Work out the finished part from the listing and answer in its coordinate system (mm). Give positions to 0.01 mm unless a question says otherwise; leave off trailing zeros. Write each loop counter-clockwise with the first axis right and the second up, starting at its lowest first coordinate (ties: lowest second). Pieces come first, ordered by that corner, then holes.
1) Given pin 1 Ø0.9 at (x, z) = (-64.5, 2) entering from +Y, flat-ended and moving along its own axis, determine where the tip first touches the part or whether it passes through.
2) Straight lines are drawn through the part: probe 1 along X at (y, z) = (17.5, 0.2); probe 2 along Y at (x, z) = (-15, 2.15); probe 3 along X at (y, z) = (-11, 1). For each, find the intervals that lie inside material, in ascending order.
3) Find section A-A (x = 8). Determine the outline of the cut face in (y, z).
4) Find section B-B (z = 1.5). Count the separate pieces of the cut face and the enclosed holes in it, plus the area to 3 significant figures.
```python
from build123d import *

# Parameters (mm, degrees)
SKETCH1_R           = 1.42
SKETCH1_W           = 25.000092503
SKETCH1_H           = 60
SKETCH1_W_2         = 30
SKETCH1_H_2         = 30
SKETCH1_W_3         = 20
SKETCH1_H_3         = 1
BOSS_EXTRUDE1_DEPTH = 3


with BuildPart() as part:
    # Sketch1 → Boss-Extrude1 (new body)
    with BuildSketch(Plane.XY):
        Polygon((-55, 45), (45, 45), (45, -45), (-55, -45), (-55, -30), (-140, -30), (-140, 30), (-55, 30), align=None)
        with Locations((15, 39)):
            Circle(SKETCH1_R, mode=Mode.SUBTRACT)
        with Locations((-15, 39)):
            Circle(SKETCH1_R, mode=Mode.SUBTRACT)
        with Locations((-15, -39)):
            Circle(SKETCH1_R, mode=Mode.SUBTRACT)
        with Locations((15, -39)):
            Circle(SKETCH1_R, mode=Mode.SUBTRACT)
        with Locations((30.000092503, 39.056338633)):
            Circle(SKETCH1_R, mode=Mode.SUBTRACT)
        with Locations((40, 39.013326424)):
            Circle(SKETCH1_R, mode=Mode.SUBTRACT)
        with Locations((-55, 20)):
            Circle(SKETCH1_R, mode=Mode.SUBTRACT)
        with Locations((-55, -20)):
            Circle(SKETCH1_R, mode=Mode.SUBTRACT)
        with Locations((40, -39.013326424)):
            Circle(SKETCH1_R, mode=Mode.SUBTRACT)
        with Locations((30.000092503, -39.056338633)):
            Circle(SKETCH1_R, mode=Mode.SUBTRACT)
        with Locations((-135, 5)):
            Circle(SKETCH1_R, mode=Mode.SUBTRACT)
        with Locations((-135, -5)):
            Circle(SKETCH1_R, mode=Mode.SUBTRACT)
        Polygon((-15, 30), (-45, 30), (-45, 15), (-85, 15), (-85, -15), (-45, -15), (-45, -30), (-5, -30), (-5, 30), align=None, mode=Mode.SUBTRACT)
        with Locations((17.500046252, 0)):
            Rectangle(SKETCH1_W, SKETCH1_H, mode=Mode.SUBTRACT)
        with Locations((-110, 0)):
            Rectangle(SKETCH1_W_2, SKETCH1_H_2, mode=Mode.SUBTRACT)
        with Locations((-110, -24.5)):
            Rectangle(SKETCH1_W_3, SKETCH1_H_3, mode=Mode.SUBTRACT)
        with Locations((-110, 24.5)):
            Rectangle(SKETCH1_W_3, SKETCH1_H_3, mode=Mode.SUBTRACT)
    extrude(amount=BOSS_EXTRUDE1_DEPTH)


solid = part.part
```
Results:
1. pin 1: stops at y = 30
2. probe 1: x = -140 to -45, -5 to 5, 30 to 45
2. probe 2: y = -45 to -40.42, -37.58 to -30, 30 to 37.58, 40.42 to 45
2. probe 3: x = -140 to -125, -95 to -85, -5 to 5, 30 to 45
3. outline: (-45, 0) - (-30, 0) - (-30, 3) - (-45, 3) - close; (30, 0) - (45, 0) - (45, 3) - (30, 3) - close
4. separate pieces: 1
4. enclosed holes: 17
4. area: 7,980 mm2
